Build history of the part. All positions in model axes, mm. Face numbers are marked on the shaded views. A direction names the side the tool comes from. Round coordinates to 2 decimals unless told otherwise and drop trailing zeros. Write each loop counter-clockwise with the first axis right and the second up, starting at its lowest first coordinate (ties: lowest second). Pieces come first, ordered by that corner, then holes.
from build123d import *

# Parameters (mm, degrees)
BOSS_EXTRUDE1_DEPTH = 31.75
SKETCH2_R           = 6.35
CUT_EXTRUDE1_DEPTH  = 58.557767504
SKETCH3_R           = 1.5
CUT_EXTRUDE2_DEPTH  = 58.557767504
BOSS_EXTRUDE2_DEPTH = 2.54
BOSS_EXTRUDE3_START = -29.21
BOSS_EXTRUDE3_DEPTH = 2.54
SKETCH5_R           = 1.75
CUT_EXTRUDE3_DEPTH  = 2.54
CHAMFER1_SIZE       = 1.5875


with BuildPart() as part:
    # Sketch1 → Boss-Extrude1 (new body)
    with BuildSketch(Plane.XY):
        Polygon((0, 0), (0, 29.21), (2.54, 29.21), (2.54, 1.5875), (38.1, 1.5875), (38.1, 0), align=None)
    extrude(amount=BOSS_EXTRUDE1_DEPTH)

    # Sketch2 → Cut-Extrude1 (cut, through all)
    with BuildSketch(Plane.ZY):
        with Locations((15.875, 16.51)):
            Circle(SKETCH2_R)
    extrude(amount=-CUT_EXTRUDE1_DEPTH, mode=Mode.SUBTRACT)

    # Sketch3 → Cut-Extrude2 (cut, through all)
    with BuildSketch(Plane.ZY):
        with Locations((6.875, 16.51)):
            Circle(SKETCH3_R)
        with BuildLine():
            ThreePointArc((21.701961434, 12.537127658), (22.225, 16.51), (21.701961434, 20.482872342))
            ThreePointArc((21.701961434, 20.482872342), (13.9248315, 24.973000403), (9.43470344, 17.19587047))
            ThreePointArc((9.43470344, 17.19587047), (9.525, 16.51), (9.43470344, 15.82412953))
            ThreePointArc((9.43470344, 15.82412953), (13.9248315, 8.046999597), (21.701961434, 12.537127658))
        make_face()
        with BuildLine():
            ThreePointArc((25.79507191, 11.440382011), (26.46249978, 16.51), (25.79507191, 21.579617989))
            ThreePointArc((25.79507191, 21.579617989), (23.850789427, 22.702150004), (22.728257411, 20.757867521))
            ThreePointArc((22.728257411, 20.757867521), (23.28749978, 16.51), (22.728257411, 12.262132479))
            ThreePointArc((22.728257411, 12.262132479), (23.850789427, 10.317849996), (25.79507191, 11.440382011))
        make_face()
    extrude(amount=-CUT_EXTRUDE2_DEPTH, mode=Mode.SUBTRACT)

    # Sketch4 → Boss-Extrude2 (add)
    with BuildSketch(Plane.XY.offset(31.75)):
        Polygon((2.54, 29.21), (30.1625, 1.5875), (2.54, 1.5875), align=None)
    extrude(amount=-BOSS_EXTRUDE2_DEPTH)

    # Sketch4<2> → Boss-Extrude3 (add)
    with BuildSketch(Plane.XY.offset(31.75).offset(BOSS_EXTRUDE3_START)):
        Polygon((2.54, 29.21), (30.1625, 1.5875), (2.54, 1.5875), align=None)
    extrude(amount=-BOSS_EXTRUDE3_DEPTH)

    # Sketch5 → Cut-Extrude3 (cut)
    with BuildSketch(Plane(origin=(0, 1.5875, 0), x_dir=(1, 0, 0), z_dir=(0, 1, 0))):
        with Locations(Location((7.62, -6.35, 0), (0, 0, 270))):
            Circle(SKETCH5_R)
        with Locations(Location((31.75, -25.4, 0), (0, 0, 270))):
            Circle(SKETCH5_R)
        with Locations(Location((31.75, -6.35, 0), (0, 0, 270))):
            Circle(SKETCH5_R)
        with Locations(Location((7.62, -25.4, 0), (0, 0, 270))):
            Circle(SKETCH5_R)
        with Locations(Location((21.59, -6.35, 0), (0, 0, 270))):
            Circle(SKETCH5_R)
        with Locations(Location((21.59, -25.4, 0), (0, 0, 270))):
            Circle(SKETCH5_R)
    extrude(amount=-CUT_EXTRUDE3_DEPTH, mode=Mode.SUBTRACT)

    # Chamfer1
    chamfer1_edges = [part.edges().sort_by_distance(p)[0] for p in [
        (31.75, 1.5875, 23.65),
        (31.75, 1.5875, 4.6),
        (7.62, 1.5875, 23.65),
        (21.59, 1.5875, 23.65),
        (21.59, 1.5875, 4.6),
        (7.62, 1.5875, 4.6),
    ]]
    chamfer(chamfer1_edges, length=CHAMFER1_SIZE - 0.0001)  # a hair under: the kernel refuses the full size


solid = part.part
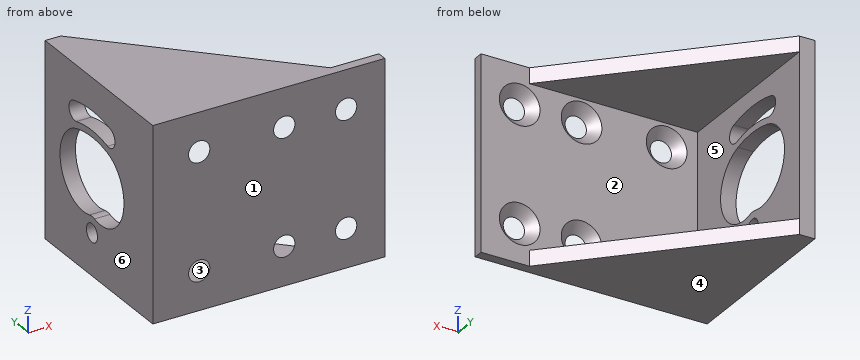
1) Slice it at D-D (x = 17). Write the cut outline in (y, z).
Results:
outline: (0, 0) - (14.75, 0) - (14.75, 2.54) - (1.59, 2.54) - (1.59, 29.21) - (14.75, 29.21) - (14.75, 31.75) - (0, 31.75) - close
2) Wall check: L1, parallel to X at y = 0.05, z = 6.35; L2, parallel to Z at x = 10, y = 18.5; L3, parallel to X at y = 12.25, z = 29. Give the ranges that are in metal, low to high.
Results:
L1: x = 0 to 5.82, 9.42 to 19.79, 23.39 to 29.95, 33.55 to 38.1
L2: z = 0 to 2.54, 29.21 to 31.75
L3: x = 0 to 2.54
3) Which spindle directions (+Z, -Z, +X, -X, +Y, -Y) get a long thin tool onto all of the face, cutting with end or side? Do the marked faces 5 and 6. Say none if no direction does.
Results:
face 5: +X, +Y
face 6: +Z, -Z, -X, +Y, -Y
4) Pin check, flat tips, straight feed: pin 1 Ø3 at (y, z) = (12, 7.5) entering from +X; pin 2 Ø4.5 at (x, z) = (31.75, 25.4) entering from -Y; pin 3 Ø5 at (x, z) = (10.5, 26.5) entering from +Y; pin 4 Ø4.5 at (x, z) = (21.59, 6.35) entering from +Y. Stop position of each tip, or through.
Results:
pin 1: stops at x = 2.54
pin 2: stops at y = 0
pin 3: stops at y = 1.59
pin 4: stops at y = 0.5
5) Mould opens along Z. For the marked faces 1, 2, 3 and 4 say: released by +Z, released by -Z, zero draft, split by the parting line, or undercut.
Results:
face 1: zero draft
face 2: undercut
face 3: undercut
face 4: released by -Z
6) Slice it at B-B (z = 14). Write the cut outline in (x, y), plus the area to 3 significant figures.
Results:
outline: (0, 0) - (38.1, 0) - (38.1, 1.59) - (2.54, 1.59) - (2.54, 8.03) - (0, 8.03) - close; (0, 24.99) - (2.54, 24.99) - (2.54, 29.21) - (0, 29.21) - close
area: 87.6 mm2
7) Slice it at A-A (x = 21.59). Count the separate pieces of the cut face and the enclosed holes in it, plus the area to 3 significant figures.
Results:
separate pieces: 3
enclosed holes: 0
area: 77.8 mm2
